The listing builds one solid part. Answer for the finished solid, in the listing's coordinates (mm). A direction names the side the tool comes from. Coordinates: 2 decimals unless noted, no trailing zeros. Write each loop counter-clockwise with the first axis right and the second up, starting at its lowest first coordinate (ties: lowest second). Pieces come first, ordered by that corner, then holes.
(1) For a pull along X with two mould halves and no side action, classify faces 1 (the cylindrical face through (-1.2, 32.9, 9)), 2 (the flat face through (42, 40, 5)), 3 (the cylindrical face through (-73, 39, 5)) as +X half, -X half, draft (parallel to the pull), parting line (faces both ways), or undercut.
(2) The part is cut by section A-A on z = 3.75. Determine the outline of the cut face in (x, y), plus the area to 3 significant figures.
(3) The part is cut by section B-B on x = 0. Determine the outline of the cut face in (y, z).
(4) Given P1, Ø2.5, axis at x = 0, y = 32, coming from the +Z side; P2, Ø5, axis at x = -53.5, z = 2.5, coming from the +Y side; P3, Ø4, axis at x = -8, y = 40, coming from the -Z side, each flat-ended and moving along its own axis, determine where each tip first touches the part or whether it passes through.
(5) Which of the six approach directions +Z, -Z, +X, -X, +Y, -Y give full straight-line access (tool end or side, diameter ignored) to faces 4 (the flat face through (-42, 40, 5)), 5 (the cylindrical face through (0, 54, 5)), 6 (the cylindrical face through (-8.11, 32.57, 3.94))?
(6) The part is cut by section C-C on y = 48. Determine the outline of the cut face in (x, z).
(7) Straight lines are drawn through the part: line 1 (Y direction, x = 0, z = 8.7); line 2 (Y direction, x = 0, z = 5.25); line 3 (Y direction, x = 64.5, z = 8). For each, find the intervals that lie inside material, in ascending order.
(8) The part is cut by section D-D on x = 38. Determine the outline of the cut face in (y, z).
Autodesk Fusion 360 part; units mm, degrees
sketch "Sketch1" plane through (0, 0, 0) normal (0, 0, 1) x (1, 0, 0)
  line L0 (75, 40) -> (-75, 40)
  line L1 (-75, 40) -> (-75, -40)
  line L2 (-75, -40) -> (75, -40)
  line L3 (75, -40) -> (75, 40)
  line L4 (75, 40) -> (-75, -40) construction
  line L5 (-75, 40) -> (75, -40) construction
  dimension "d1" = 150
  dimension "d2" = 80
extrude "Extrude1" add sketch "Sketch1" along normal blind 10
sketch "Sketch2" plane through (0, 0, 0) normal (0, 0, 1) x (1, 0, 0)
  circle A0 centre (0, 40) radius 14
  dimension "d10" = 28
extrude "Extrude2" add sketch "Sketch2" along normal blind 10
sketch "Sketch3" plane through (0, 0, 0) normal (0, 0, 1) x (1, 0, 0)
  circle A0 centre (0, 40) radius 11
  dimension "d7" = 22
extrude "Extrude3" cut sketch "Sketch3" along normal blind 8
fillet "Fillet1" radius 5 4 edges at (75, -40, 5) (75, 40, 5) (-75, -40, 5) (-75, 40, 5)
sketch "Sketch4" plane through (0, 0, 8) normal (0, 0, -1) x (1, 0, 0)
  circle A0 centre (0, -32) radius 1.5
  circle A1 centre (0, -48) radius 1.5
  circle A2 centre (-8, -40) radius 1.5
  circle A3 centre (8, -40) radius 1.5
  circle A4 centre (0, -40) radius 11
  dimension "d13" = 3
  dimension "d14" = 3
  dimension "d15" = 3
  dimension "d16" = 3
extrude "Extrude4" cut sketch "Sketch4" against normal blind 2 contours A0 | A1 | A2 | A3
Model answer:
1. face 1: undercut
1. face 2: draft
1. face 3: -X half
2. outline: (-75, -35) arc R5 ccw to (-70, -40) - (70, -40) arc R5 ccw to (75, -35) - (75, 35) arc R5 ccw to (70, 40) - (14, 40) arc R14 ccw to (-14, 40) - (-70, 40) arc R5 ccw to (-75, 35) - close; hole circle Ø22 at (0, 40)
2. area: 11,900 mm2
3. outline: (-40, 0) - (29, 0) - (29, 8) - (30.5, 8) - (30.5, 10) - (-40, 10) - close; (33.5, 8) - (46.5, 8) - (46.5, 10) - (33.5, 10) - close; (49.5, 8) - (51, 8) - (51, 0) - (54, 0) - (54, 10) - (49.5, 10) - close
4. P1: passes through
4. P2: stops at y = 40
4. P3: stops at z = 8
5. face 4: +Z, -Z, -X, +Y
5. face 5: +Z, -Z, +Y
5. face 6: -Z
6. outline: (-11.49, 0) - (-7.55, 0) - (-7.55, 8) - (-1.5, 8) - (-1.5, 10) - (-11.49, 10) - close; (1.5, 8) - (7.55, 8) - (7.55, 0) - (11.49, 0) - (11.49, 10) - (1.5, 10) - close
7. line 1: y = -40 to 30.5, 33.5 to 46.5, 49.5 to 54
7. line 2: y = -40 to 29, 51 to 54
7. line 3: y = -40 to 40
8. outline: (-40, 0) - (40, 0) - (40, 10) - (-40, 10) - close
